```python
from build123d import *

# Parameters (mm, degrees)
SKETCH_1_W          = 350
SKETCH_1_H          = 20
SKETCH_1_W_2        = 20
SKETCH_1_H_2        = 310
SKETCH_1_W_3        = 100
EXTRUDE_1_DEPTH     = 20
CUT_EXTRUDE_1_REACH = 424.404
SKETCH_2_R          = 1.75
SKETCH_3_W          = 20
SKETCH_3_H          = 20
EXTRUDE_2_DEPTH     = 135
SKETCH_4_R          = 1.75
CUT_EXTRUDE_2_DEPTH = 20
CUT_EXTRUDE_3_REACH = 455.211
SKETCH_5_R          = 1.75
CUT_EXTRUDE_4_REACH = 455.211
SKETCH_6_R          = 1.75
SKETCH_7_R          = 1.75
CUT_EXTRUDE_5_DEPTH = 20
SKETCH_8_R          = 1.75
CUT_EXTRUDE_6_DEPTH = 20


with BuildPart() as part:
    # 草图1 → 凸台-拉伸1 (new body)
    with BuildSketch(Plane(origin=(0, 0, 0), x_dir=(1, 0, 0), z_dir=(0, 1, 0))):
        Rectangle(SKETCH_1_W, SKETCH_1_H)
        with Locations((-165, -165)):
            Rectangle(SKETCH_1_W_2, SKETCH_1_H_2)
        with Locations((165, -165)):
            Rectangle(SKETCH_1_W_2, SKETCH_1_H_2)
        with Locations((-225, 0)):
            Rectangle(SKETCH_1_W_3, SKETCH_1_H)
    extrude(amount=EXTRUDE_1_DEPTH)

    # 草图2 → 切除-拉伸1 (cut, up to next)
    with BuildSketch(Plane(origin=(0, 20, 0), x_dir=(1, 0, 0), z_dir=(0, 1, 0)), mode=Mode.PRIVATE) as cut_extrude_1_sk1:
        with Locations(Location((-145, 0, 0), (0, 0, 270))):
            Circle(SKETCH_2_R)
    cut_extrude_1_tool1 = extrude(cut_extrude_1_sk1.sketch, amount=-CUT_EXTRUDE_1_REACH, mode=Mode.PRIVATE) & part.part
    # 草图2 → 切除-拉伸1 (cut, up to next)
    with BuildSketch(Plane(origin=(0, 20, 0), x_dir=(1, 0, 0), z_dir=(0, 1, 0)), mode=Mode.PRIVATE) as cut_extrude_1_sk2:
        with Locations(Location((-125, 0, 0), (0, 0, 270))):
            Circle(SKETCH_2_R)
    cut_extrude_1_tool2 = extrude(cut_extrude_1_sk2.sketch, amount=-CUT_EXTRUDE_1_REACH, mode=Mode.PRIVATE) & part.part
    # 草图2 → 切除-拉伸1 (cut, up to next)
    with BuildSketch(Plane(origin=(0, 20, 0), x_dir=(1, 0, 0), z_dir=(0, 1, 0)), mode=Mode.PRIVATE) as cut_extrude_1_sk3:
        with Locations(Location((-165, -310, 0), (0, 0, 270))):
            Circle(SKETCH_2_R)
    cut_extrude_1_tool3 = extrude(cut_extrude_1_sk3.sketch, amount=-CUT_EXTRUDE_1_REACH, mode=Mode.PRIVATE) & part.part
    # 草图2 → 切除-拉伸1 (cut, up to next)
    with BuildSketch(Plane(origin=(0, 20, 0), x_dir=(1, 0, 0), z_dir=(0, 1, 0)), mode=Mode.PRIVATE) as cut_extrude_1_sk4:
        with Locations(Location((125, 0, 0), (0, 0, 270))):
            Circle(SKETCH_2_R)
    cut_extrude_1_tool4 = extrude(cut_extrude_1_sk4.sketch, amount=-CUT_EXTRUDE_1_REACH, mode=Mode.PRIVATE) & part.part
    # 草图2 → 切除-拉伸1 (cut, up to next)
    with BuildSketch(Plane(origin=(0, 20, 0), x_dir=(1, 0, 0), z_dir=(0, 1, 0)), mode=Mode.PRIVATE) as cut_extrude_1_sk5:
        with Locations(Location((145, 0, 0), (0, 0, 270))):
            Circle(SKETCH_2_R)
    cut_extrude_1_tool5 = extrude(cut_extrude_1_sk5.sketch, amount=-CUT_EXTRUDE_1_REACH, mode=Mode.PRIVATE) & part.part
    # 草图2 → 切除-拉伸1 (cut, up to next)
    with BuildSketch(Plane(origin=(0, 20, 0), x_dir=(1, 0, 0), z_dir=(0, 1, 0)), mode=Mode.PRIVATE) as cut_extrude_1_sk6:
        with Locations(Location((165, 0, 0), (0, 0, 270))):
            Circle(SKETCH_2_R)
    cut_extrude_1_tool6 = extrude(cut_extrude_1_sk6.sketch, amount=-CUT_EXTRUDE_1_REACH, mode=Mode.PRIVATE) & part.part
    # 草图2 → 切除-拉伸1 (cut, up to next)
    with BuildSketch(Plane(origin=(0, 20, 0), x_dir=(1, 0, 0), z_dir=(0, 1, 0)), mode=Mode.PRIVATE) as cut_extrude_1_sk7:
        with Locations(Location((165, -20, 0), (0, 0, 270))):
            Circle(SKETCH_2_R)
    cut_extrude_1_tool7 = extrude(cut_extrude_1_sk7.sketch, amount=-CUT_EXTRUDE_1_REACH, mode=Mode.PRIVATE) & part.part
    # 草图2 → 切除-拉伸1 (cut, up to next)
    with BuildSketch(Plane(origin=(0, 20, 0), x_dir=(1, 0, 0), z_dir=(0, 1, 0)), mode=Mode.PRIVATE) as cut_extrude_1_sk8:
        with Locations(Location((165, -290, 0), (0, 0, 270))):
            Circle(SKETCH_2_R)
    cut_extrude_1_tool8 = extrude(cut_extrude_1_sk8.sketch, amount=-CUT_EXTRUDE_1_REACH, mode=Mode.PRIVATE) & part.part
    # 草图2 → 切除-拉伸1 (cut, up to next)
    with BuildSketch(Plane(origin=(0, 20, 0), x_dir=(1, 0, 0), z_dir=(0, 1, 0)), mode=Mode.PRIVATE) as cut_extrude_1_sk9:
        with Locations(Location((165, -310, 0), (0, 0, 270))):
            Circle(SKETCH_2_R)
    cut_extrude_1_tool9 = extrude(cut_extrude_1_sk9.sketch, amount=-CUT_EXTRUDE_1_REACH, mode=Mode.PRIVATE) & part.part
    # 草图2 → 切除-拉伸1 (cut, up to next)
    with BuildSketch(Plane(origin=(0, 20, 0), x_dir=(1, 0, 0), z_dir=(0, 1, 0)), mode=Mode.PRIVATE) as cut_extrude_1_sk10:
        with Locations(Location((-105, 0, 0), (0, 0, 270))):
            Circle(SKETCH_2_R)
    cut_extrude_1_tool10 = extrude(cut_extrude_1_sk10.sketch, amount=-CUT_EXTRUDE_1_REACH, mode=Mode.PRIVATE) & part.part
    # 草图2 → 切除-拉伸1 (cut, up to next)
    with BuildSketch(Plane(origin=(0, 20, 0), x_dir=(1, 0, 0), z_dir=(0, 1, 0)), mode=Mode.PRIVATE) as cut_extrude_1_sk11:
        with Locations(Location((-165, 0, 0), (0, 0, 270))):
            Circle(SKETCH_2_R)
    cut_extrude_1_tool11 = extrude(cut_extrude_1_sk11.sketch, amount=-CUT_EXTRUDE_1_REACH, mode=Mode.PRIVATE) & part.part
    # 草图2 → 切除-拉伸1 (cut, up to next)
    with BuildSketch(Plane(origin=(0, 20, 0), x_dir=(1, 0, 0), z_dir=(0, 1, 0)), mode=Mode.PRIVATE) as cut_extrude_1_sk12:
        with Locations(Location((-165, -20, 0), (0, 0, 270))):
            Circle(SKETCH_2_R)
    cut_extrude_1_tool12 = extrude(cut_extrude_1_sk12.sketch, amount=-CUT_EXTRUDE_1_REACH, mode=Mode.PRIVATE) & part.part
    # 草图2 → 切除-拉伸1 (cut, up to next)
    with BuildSketch(Plane(origin=(0, 20, 0), x_dir=(1, 0, 0), z_dir=(0, 1, 0)), mode=Mode.PRIVATE) as cut_extrude_1_sk13:
        with Locations(Location((-165, -290, 0), (0, 0, 270))):
            Circle(SKETCH_2_R)
    cut_extrude_1_tool13 = extrude(cut_extrude_1_sk13.sketch, amount=-CUT_EXTRUDE_1_REACH, mode=Mode.PRIVATE) & part.part
    # 草图2 → 切除-拉伸1 (cut, up to next)
    with BuildSketch(Plane(origin=(0, 20, 0), x_dir=(1, 0, 0), z_dir=(0, 1, 0)), mode=Mode.PRIVATE) as cut_extrude_1_sk14:
        with Locations(Location((-185, 0, 0), (0, 0, 270))):
            Circle(SKETCH_2_R)
    cut_extrude_1_tool14 = extrude(cut_extrude_1_sk14.sketch, amount=-CUT_EXTRUDE_1_REACH, mode=Mode.PRIVATE) & part.part
    # 草图2 → 切除-拉伸1 (cut, up to next)
    with BuildSketch(Plane(origin=(0, 20, 0), x_dir=(1, 0, 0), z_dir=(0, 1, 0)), mode=Mode.PRIVATE) as cut_extrude_1_sk15:
        with Locations(Location((-165, -40, 0), (0, 0, 270))):
            Circle(SKETCH_2_R)
    cut_extrude_1_tool15 = extrude(cut_extrude_1_sk15.sketch, amount=-CUT_EXTRUDE_1_REACH, mode=Mode.PRIVATE) & part.part
    add(cut_extrude_1_tool1.solids().sort_by_distance((-145, 20, 0))[0], mode=Mode.SUBTRACT)
    add(cut_extrude_1_tool2.solids().sort_by_distance((-125, 20, 0))[0], mode=Mode.SUBTRACT)
    add(cut_extrude_1_tool3.solids().sort_by_distance((-165, 20, 310))[0], mode=Mode.SUBTRACT)
    add(cut_extrude_1_tool4.solids().sort_by_distance((125, 20, 0))[0], mode=Mode.SUBTRACT)
    add(cut_extrude_1_tool5.solids().sort_by_distance((145, 20, 0))[0], mode=Mode.SUBTRACT)
    add(cut_extrude_1_tool6.solids().sort_by_distance((165, 20, 0))[0], mode=Mode.SUBTRACT)
    add(cut_extrude_1_tool7.solids().sort_by_distance((165, 20, 20))[0], mode=Mode.SUBTRACT)
    add(cut_extrude_1_tool8.solids().sort_by_distance((165, 20, 290))[0], mode=Mode.SUBTRACT)
    add(cut_extrude_1_tool9.solids().sort_by_distance((165, 20, 310))[0], mode=Mode.SUBTRACT)
    add(cut_extrude_1_tool10.solids().sort_by_distance((-105, 20, 0))[0], mode=Mode.SUBTRACT)
    add(cut_extrude_1_tool11.solids().sort_by_distance((-165, 20, 0))[0], mode=Mode.SUBTRACT)
    add(cut_extrude_1_tool12.solids().sort_by_distance((-165, 20, 20))[0], mode=Mode.SUBTRACT)
    add(cut_extrude_1_tool13.solids().sort_by_distance((-165, 20, 290))[0], mode=Mode.SUBTRACT)
    add(cut_extrude_1_tool14.solids().sort_by_distance((-185, 20, 0))[0], mode=Mode.SUBTRACT)
    add(cut_extrude_1_tool15.solids().sort_by_distance((-165, 20, 40))[0], mode=Mode.SUBTRACT)

    # 草图3 → 凸台-拉伸2 (add)
    with BuildSketch(Plane(origin=(175, 0, 0), x_dir=(0, 0, -1), z_dir=(1, 0, 0))):
        with Locations((0, 10)):
            Rectangle(SKETCH_3_W, SKETCH_3_H)
    extrude(amount=EXTRUDE_2_DEPTH)

    # 草图4 → 切除-拉伸2 (cut)
    with BuildSketch(Plane(origin=(0, 20, 0), x_dir=(1, 0, 0), z_dir=(0, 1, 0))):
        with Locations(Location((165, -40, 0), (0, 0, 270))):
            Circle(SKETCH_4_R)
        with Locations(Location((185, 0, 0), (0, 0, 270))):
            Circle(SKETCH_4_R)
    extrude(amount=-CUT_EXTRUDE_2_DEPTH, mode=Mode.SUBTRACT)

    # 草图5 → 切除-拉伸3 (cut, up to next)
    with BuildSketch(Plane(origin=(0, 0, -10), x_dir=(-1, 0, 0), z_dir=(0, 0, -1)), mode=Mode.PRIVATE) as cut_extrude_3_sk1:
        with Locations((40, 10)):
            Circle(SKETCH_5_R)
    cut_extrude_3_tool1 = extrude(cut_extrude_3_sk1.sketch, amount=-CUT_EXTRUDE_3_REACH, mode=Mode.PRIVATE) & part.part
    # 草图5 → 切除-拉伸3 (cut, up to next)
    with BuildSketch(Plane(origin=(0, 0, -10), x_dir=(-1, 0, 0), z_dir=(0, 0, -1)), mode=Mode.PRIVATE) as cut_extrude_3_sk2:
        with Locations((20, 10)):
            Circle(SKETCH_5_R)
    cut_extrude_3_tool2 = extrude(cut_extrude_3_sk2.sketch, amount=-CUT_EXTRUDE_3_REACH, mode=Mode.PRIVATE) & part.part
    # 草图5 → 切除-拉伸3 (cut, up to next)
    with BuildSketch(Plane(origin=(0, 0, -10), x_dir=(-1, 0, 0), z_dir=(0, 0, -1)), mode=Mode.PRIVATE) as cut_extrude_3_sk3:
        with Locations((0, 10)):
            Circle(SKETCH_5_R)
    cut_extrude_3_tool3 = extrude(cut_extrude_3_sk3.sketch, amount=-CUT_EXTRUDE_3_REACH, mode=Mode.PRIVATE) & part.part
    add(cut_extrude_3_tool1.solids().sort_by_distance((-40, 10, -10))[0], mode=Mode.SUBTRACT)
    add(cut_extrude_3_tool2.solids().sort_by_distance((-20, 10, -10))[0], mode=Mode.SUBTRACT)
    add(cut_extrude_3_tool3.solids().sort_by_distance((0, 10, -10))[0], mode=Mode.SUBTRACT)

    # 草图6 → 切除-拉伸4 (cut, up to next)
    with BuildSketch(Plane(origin=(0, 0, -10), x_dir=(-1, 0, 0), z_dir=(0, 0, -1)), mode=Mode.PRIVATE) as cut_extrude_4_sk1:
        with Locations((-300, 10)):
            Circle(SKETCH_6_R)
    cut_extrude_4_tool1 = extrude(cut_extrude_4_sk1.sketch, amount=-CUT_EXTRUDE_4_REACH, mode=Mode.PRIVATE) & part.part
    # 草图6 → 切除-拉伸4 (cut, up to next)
    with BuildSketch(Plane(origin=(0, 0, -10), x_dir=(-1, 0, 0), z_dir=(0, 0, -1)), mode=Mode.PRIVATE) as cut_extrude_4_sk2:
        with Locations((-280, 10)):
            Circle(SKETCH_6_R)
    cut_extrude_4_tool2 = extrude(cut_extrude_4_sk2.sketch, amount=-CUT_EXTRUDE_4_REACH, mode=Mode.PRIVATE) & part.part
    add(cut_extrude_4_tool1.solids().sort_by_distance((300, 10, -10))[0], mode=Mode.SUBTRACT)
    add(cut_extrude_4_tool2.solids().sort_by_distance((280, 10, -10))[0], mode=Mode.SUBTRACT)

    # 草图7 → 切除-拉伸5 (cut)
    with BuildSketch(Plane(origin=(0, 0, -10), x_dir=(-1, 0, 0), z_dir=(0, 0, -1))):
        with Locations((-80, 10)):
            Circle(SKETCH_7_R)
        with Locations((-60, 10)):
            Circle(SKETCH_7_R)
    extrude(amount=-CUT_EXTRUDE_5_DEPTH, mode=Mode.SUBTRACT)

    # 草图8 → 切除-拉伸6 (cut)
    with BuildSketch(Plane.XZ):
        with Locations(Location((-60, 0, 0), (0, 0, 270))):
            Circle(SKETCH_8_R)
        with Locations(Location((-40, 0, 0), (0, 0, 270))):
            Circle(SKETCH_8_R)
        with Locations(Location((-20, 0, 0), (0, 0, 270))):
            Circle(SKETCH_8_R)
        with Locations(Location((0, 0, 0), (0, 0, 270))):
            Circle(SKETCH_8_R)
        with Locations(Location((290, 0, 0), (0, 0, 270))):
            Circle(SKETCH_8_R)
        with Locations(Location((270, 0, 0), (0, 0, 270))):
            Circle(SKETCH_8_R)
        with Locations(Location((-265, 0, 0), (0, 0, 270))):
            Circle(SKETCH_8_R)
        with Locations(Location((-245, 0, 0), (0, 0, 270))):
            Circle(SKETCH_8_R)
        with Locations(Location((-225, 0, 0), (0, 0, 270))):
            Circle(SKETCH_8_R)
    extrude(amount=-CUT_EXTRUDE_6_DEPTH, mode=Mode.SUBTRACT)


solid = part.part
```
Geometry check sheet. Reference: the model listing, model coordinates, mm. A direction names the side the tool comes from. Round coordinates to 2 decimals unless told otherwise and drop trailing zeros. Loops run counter-clockwise (first coordinate to the right, second up) from the corner with the lowest first, then second, coordinate; pieces in that order, holes last. Notation, with made-up numbers: (37, 77) -> (72, 77) arc R18 cw to (72, 103) -> close; hole circle Ø5 at (47.5, 4.25). An arc over 180 degrees is marked (long way). Use a Markdown table: item, result.
(1) Scan lines: probe 1 along Z at (x, y) = (-165, 12.75); probe 2 along X at (y, z) = (7.5, 76.5); probe 3 along Z at (x, y) = (-185.5, 6.75). Record each from-to range of solid material in increasing order.
Calculated:
| item | result |
|---|---|
| probe 1 | -10 to -1.75, 1.75 to 18.25, 21.75 to 38.25, 41.75 to 288.25, 291.75 to 308.25, 311.75 to 320 |
| probe 2 | -175 to -155, 155 to 175 |
| probe 3 | -10 to -1.68, 1.68 to 10 |
(2) Sectioned sample at B-B (y = 3.25). Give the number of separate pieces and of enclosed holes in the cut face, then the cut area to 3 significant figures.
Calculated:
| item | result |
|---|---|
| separate pieces | 1 |
| enclosed holes | 26 |
| area | 23,800 mm² |
(3) Sectioned sample at A-A (z = 194). Enter the section's corners in (x, y), then the cut area to 3 significant figures.
Calculated:
| item | result |
|---|---|
| outline | (-175, 0) -> (-155, 0) -> (-155, 20) -> (-175, 20) -> close; (155, 0) -> (175, 0) -> (175, 20) -> (155, 20) -> close |
| area | 800 mm² |
(4) Set-up check for faces 1 (the flat face through (16, 0, 9)), 2 (the flat face through (-226, 10, 10)), 3 (the flat face through (155, 10, 167)), 4 (the flat face through (175, 10, 167)): record each of +Z, -Z, +X, -X, +Y, -Y from which the full face is reachable in a straight line by a thin tool's end or side.
Calculated:
| item | result |
|---|---|
| face 1 | +Z, -Z, +X, -X, -Y |
| face 2 | +Z, -X, +Y, -Y |
| face 3 | +Z, +Y, -Y |
| face 4 | +Z, +X, +Y, -Y |
(5) Go/stop test with flat-tipped pins: P1, Ø3, axis at x = 165, z = 310, coming from the +Y side; P2, Ø10, axis at x = -35, y = 12.5, coming from the +Z side; P3, Ø5, axis at y = 12.5, z = 168, coming from the -X side. Record where each tip stops, or that it passes through.
Calculated:
| item | result |
|---|---|
| P1 | through |
| P2 | z = 10 |
| P3 | x = -175 |
(6) Sectioned sample at C-C (x = 208.5). Enter the section's corners in (y, z).
Calculated:
| item | result |
|---|---|
| outline | (0, -10) -> (20, -10) -> (20, 10) -> (0, 10) -> close |
